```python
from build123d import *

# Parameters (mm, degrees)
SKETCH_1_W           = 67.5
SKETCH_1_H           = 62.5
EXTRUDE_1_DEPTH      = 1.6
SKETCH_2_R           = 1.65
CUT_EXTRUDE_1_DEPTH  = 10
CHAMFER_1_SIZE       = 3
SKETCH_3_R           = 1.65
EXTRUDE_2_DEPTH      = 4
SKETCH_4_R           = 4
CUT_EXTRUDE_2_DEPTH  = 0.8
SKETCH_5_R           = 4.5
EXTRUDE_3_DEPTH      = 6
EXTRUDE_4_DEPTH      = 8
EXTRUDE_5_DEPTH      = 2
CUT_EXTRUDE_4_DEPTH  = 8
EXTRUDE_6_DEPTH      = 2
EXTRUDE_6_DEPTH_BACK = 2
SKETCH_10_R          = 4.5
SKETCH_10_R_2        = 1.65


with BuildPart() as part:
    # 草图1 → 凸台-拉伸1 (new body)
    with BuildSketch(Plane.XY):
        Rectangle(SKETCH_1_W, SKETCH_1_H)
    extrude(amount=EXTRUDE_1_DEPTH)

    # 草图2 → 切除-拉伸1 (cut)
    with BuildSketch(Plane.XY.offset(1.6)):
        with Locations((-22.5, 20)):
            Circle(SKETCH_2_R)
        with Locations((22.5, 20)):
            Circle(SKETCH_2_R)
        with Locations((22.5, -20)):
            Circle(SKETCH_2_R)
        with Locations((-22.5, -20)):
            Circle(SKETCH_2_R)
        Polygon((-30.75, 11.25), (-30.75, -11.25), (-33.75, -14.25), (-33.75, 14.25), align=None)
        Polygon((30.75, 11.25), (30.75, -11.25), (33.75, -14.25), (33.75, 14.25), align=None)
    extrude(amount=-CUT_EXTRUDE_1_DEPTH, mode=Mode.SUBTRACT)

    # 倒角1
    chamfer_1_edges = [part.edges().sort_by_distance(p)[0] for p in [
        (33.75, -31.25, 0.8),
        (-33.75, -31.25, 0.8),
        (-33.75, 31.25, 0.8),
        (33.75, 31.25, 0.8),
    ]]
    chamfer(chamfer_1_edges, length=CHAMFER_1_SIZE)

    # 草图3 → 凸台-拉伸2 (add)
    # profile 1 of 4: a face of its own
    with BuildSketch(Plane(origin=(0, 0, 0), x_dir=(-1, 0, 0), z_dir=(0, 0, -1))):
        Polygon((-19.901923789, 20), (-21.200961894, 22.25), (-23.799038106, 22.25), (-25.098076211, 20), (-23.799038106, 17.75), (-21.200961894, 17.75), align=None)
        with Locations(Location((-22.5, 20, 0), (0, 0, 180))):
            Circle(SKETCH_3_R, mode=Mode.SUBTRACT)
    # profile 2 of 4: a face of its own
    with BuildSketch(Plane(origin=(0, 0, 0), x_dir=(-1, 0, 0), z_dir=(0, 0, -1))):
        Polygon((25.098076211, 20), (23.799038106, 22.25), (21.200961894, 22.25), (19.901923789, 20), (21.200961894, 17.75), (23.799038106, 17.75), align=None)
        with Locations(Location((22.5, 20, 0), (0, 0, 180))):
            Circle(SKETCH_3_R, mode=Mode.SUBTRACT)
    # profile 3 of 4: a face of its own
    with BuildSketch(Plane(origin=(0, 0, 0), x_dir=(-1, 0, 0), z_dir=(0, 0, -1))):
        Polygon((25.098076211, -20), (23.799038106, -17.75), (21.200961894, -17.75), (19.901923789, -20), (21.200961894, -22.25), (23.799038106, -22.25), align=None)
        with Locations(Location((22.5, -20, 0), (0, 0, 180))):
            Circle(SKETCH_3_R, mode=Mode.SUBTRACT)
    # profile 4 of 4: a face of its own
    with BuildSketch(Plane(origin=(0, 0, 0), x_dir=(-1, 0, 0), z_dir=(0, 0, -1))):
        Polygon((-19.901923789, -20), (-21.200961894, -17.75), (-23.799038106, -17.75), (-25.098076211, -20), (-23.799038106, -22.25), (-21.200961894, -22.25), align=None)
        with Locations(Location((-22.5, -20, 0), (0, 0, 180))):
            Circle(SKETCH_3_R, mode=Mode.SUBTRACT)
    extrude(amount=EXTRUDE_2_DEPTH)

    # 草图4 → 切除-拉伸2 (cut)
    with BuildSketch(Plane.XY.offset(1.6)):
        with Locations((-22.5, 20)):
            Circle(SKETCH_4_R)
        with Locations((22.5, 20)):
            Circle(SKETCH_4_R)
        with Locations((22.5, -20)):
            Circle(SKETCH_4_R)
        with Locations((-22.5, -20)):
            Circle(SKETCH_4_R)
    extrude(amount=-CUT_EXTRUDE_2_DEPTH, mode=Mode.SUBTRACT)

    # 草图5 → 凸台-拉伸3 (add)
    # profile 1 of 4: a face of its own
    with BuildSketch(Plane(origin=(0, 0, 0), x_dir=(-1, 0, 0), z_dir=(0, 0, -1))):
        with Locations(Location((-22.5, 20, 0), (0, 0, 180))):
            Circle(SKETCH_5_R)
        Polygon((-21.200961894, 17.75), (-19.901923789, 20), (-21.200961894, 22.25), (-23.799038106, 22.25), (-25.098076211, 20), (-23.799038106, 17.75), align=None, mode=Mode.SUBTRACT)
    # profile 2 of 4: a face of its own
    with BuildSketch(Plane(origin=(0, 0, 0), x_dir=(-1, 0, 0), z_dir=(0, 0, -1))):
        with Locations(Location((22.5, 20, 0), (0, 0, 180))):
            Circle(SKETCH_5_R)
        Polygon((23.799038106, 17.75), (25.098076211, 20), (23.799038106, 22.25), (21.200961894, 22.25), (19.901923789, 20), (21.200961894, 17.75), align=None, mode=Mode.SUBTRACT)
    # profile 3 of 4: a face of its own
    with BuildSketch(Plane(origin=(0, 0, 0), x_dir=(-1, 0, 0), z_dir=(0, 0, -1))):
        with Locations(Location((22.5, -20, 0), (0, 0, 180))):
            Circle(SKETCH_5_R)
        Polygon((23.799038106, -22.25), (25.098076211, -20), (23.799038106, -17.75), (21.200961894, -17.75), (19.901923789, -20), (21.200961894, -22.25), align=None, mode=Mode.SUBTRACT)
    # profile 4 of 4: a face of its own
    with BuildSketch(Plane(origin=(0, 0, 0), x_dir=(-1, 0, 0), z_dir=(0, 0, -1))):
        with Locations(Location((-22.5, -20, 0), (0, 0, 180))):
            Circle(SKETCH_5_R)
        Polygon((-21.200961894, -22.25), (-19.901923789, -20), (-21.200961894, -17.75), (-23.799038106, -17.75), (-25.098076211, -20), (-23.799038106, -22.25), align=None, mode=Mode.SUBTRACT)
    extrude(amount=EXTRUDE_3_DEPTH)

    # 草图6 → 凸台-拉伸4 (add)
    with BuildSketch(Plane(origin=(0, 0, 0), x_dir=(-1, 0, 0), z_dir=(0, 0, -1))):
        Polygon((-30.75, -31.25), (30.75, -31.25), (33.75, -28.25), (33.75, -14.25), (30.75, -11.25), (30.75, 11.25), (33.75, 14.25), (33.75, 28.25), (30.75, 31.25), (-30.75, 31.25), (-33.75, 28.25), (-33.75, 14.25), (-30.75, 11.25), (-30.75, -11.25), (-33.75, -14.25), (-33.75, -28.25), align=None)
        Polygon((-30.335786438, -30.25), (30.335786438, -30.25), (32.75, -27.835786438), (32.75, -14.664213562), (29.75, -11.664213562), (29.75, 11.664213562), (32.75, 14.664213562), (32.75, 27.835786438), (30.335786438, 30.25), (-30.335786438, 30.25), (-32.75, 27.835786438), (-32.75, 14.664213562), (-29.75, 11.664213562), (-29.75, -11.664213562), (-32.75, -14.664213562), (-32.75, -27.835786438), align=None, mode=Mode.SUBTRACT)
    extrude(amount=EXTRUDE_4_DEPTH)

    # 草图8 → 凸台-拉伸5 (add)
    with BuildSketch(Plane(origin=(0, 0, 0), x_dir=(-1, 0, 0), z_dir=(0, 0, -1))):
        with BuildLine():
            Line((-1.5, -11.14955156), (-1.5, -12.157816416))
            ThreePointArc((-1.5, -12.157816416), (0, 12.25), (1.5, -12.157816416))
            Line((1.5, -12.157816416), (1.5, -11.14955156))
            ThreePointArc((1.5, -11.14955156), (0, 11.25), (-1.5, -11.14955156))
        make_face()
    extrude(amount=EXTRUDE_5_DEPTH)

    # 草图9 → 切除-拉伸4 (cut)
    with BuildSketch(Plane(origin=(0, 0, -8), x_dir=(-1, 0, 0), z_dir=(0, 0, -1))):
        Polygon((29.75, 11.664213562), (32.335786438, 14.25), (33.042893219, 13.542893219), (30.75, 11.25), (30.75, -11.25), (33.042893219, -13.542893219), (32.335786438, -14.25), (29.75, -11.664213562), align=None)
        Polygon((-33.042893219, 13.542893219), (-32.335786438, 14.25), (-29.75, 11.664213562), (-29.75, -11.664213562), (-32.335786438, -14.25), (-33.042893219, -13.542893219), (-30.75, -11.25), (-30.75, 11.25), align=None)
    extrude(amount=-CUT_EXTRUDE_4_DEPTH, mode=Mode.SUBTRACT)

    # 草图10 → 凸台-拉伸6 (add, two sides: drawn at the far end of the back side and taken through both)
    # profile 1 of 4: a face of its own
    with BuildSketch(Plane(origin=(0, 0, -6), x_dir=(-1, 0, 0), z_dir=(0, 0, -1)).offset(-EXTRUDE_6_DEPTH_BACK)):
        with Locations(Location((-22.5, -20, 0), (0, 0, 180))):
            Circle(SKETCH_10_R)
        with Locations(Location((-22.5, -20, 0), (0, 0, 180))):
            Circle(SKETCH_10_R_2, mode=Mode.SUBTRACT)
    # profile 2 of 4: a face of its own
    with BuildSketch(Plane(origin=(0, 0, -6), x_dir=(-1, 0, 0), z_dir=(0, 0, -1)).offset(-EXTRUDE_6_DEPTH_BACK)):
        with Locations(Location((22.5, 20, 0), (0, 0, 180))):
            Circle(SKETCH_10_R)
        with Locations(Location((22.5, 20, 0), (0, 0, 180))):
            Circle(SKETCH_10_R_2, mode=Mode.SUBTRACT)
    # profile 3 of 4: a face of its own
    with BuildSketch(Plane(origin=(0, 0, -6), x_dir=(-1, 0, 0), z_dir=(0, 0, -1)).offset(-EXTRUDE_6_DEPTH_BACK)):
        with Locations(Location((-22.5, 20, 0), (0, 0, 180))):
            Circle(SKETCH_10_R)
        with Locations(Location((-22.5, 20, 0), (0, 0, 180))):
            Circle(SKETCH_10_R_2, mode=Mode.SUBTRACT)
    # profile 4 of 4: a face of its own
    with BuildSketch(Plane(origin=(0, 0, -6), x_dir=(-1, 0, 0), z_dir=(0, 0, -1)).offset(-EXTRUDE_6_DEPTH_BACK)):
        with Locations(Location((22.5, -20, 0), (0, 0, 180))):
            Circle(SKETCH_10_R)
        with Locations(Location((22.5, -20, 0), (0, 0, 180))):
            Circle(SKETCH_10_R_2, mode=Mode.SUBTRACT)
    extrude(amount=EXTRUDE_6_DEPTH + EXTRUDE_6_DEPTH_BACK)


solid = part.part
```
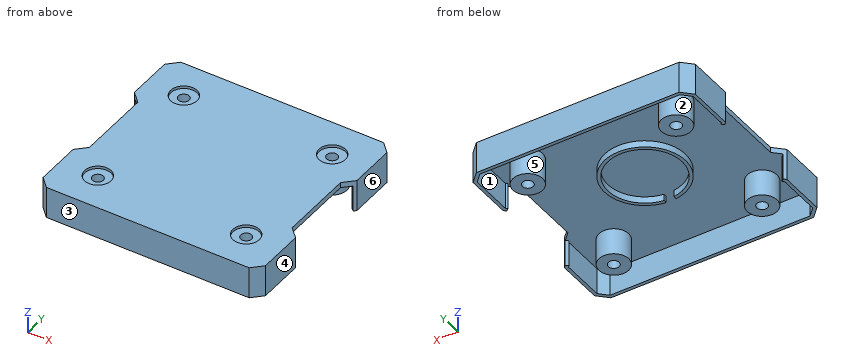
Design review of the part built by this model. Coordinates are the model's own, in mm. Face numbers are marked on the shaded views. A direction names the side the tool comes from. Coordinates: 2 decimals unless noted, no trailing zeros. Write each loop counter-clockwise with the first axis right and the second up, starting at its lowest first coordinate (ties: lowest second). Pieces come first, ordered by that corner, then holes.
1) Insertion check: pin 1 (0.8 mm diameter, centred on y = -11.5, z = -0.5, fed in from +X); pin 2 (18 mm diameter, centred on x = 0, y = 0, fed in from -Z); pin 3 (6.5 mm diameter, centred on x = 22.5, y = 20.5, fed in from +Z); pin 4 (9 mm diameter, centred on x = 23.5, y = -18.5, fed in from +Z). Each pin has a flat end and moves straight along its axis. Give the tip position at first contact, or say it passes through.
2) To check wall thickness, follow L1, parallel to Y at x = 22.5, z = 1.15; L2, parallel to X at y = -20, z = -6.25; L3, parallel to Y at x = -22.5, z = -5.25. State the ranges of each line that lie inside material, in increasing order.
3) Mouldability with a two-part tool opening along X and no side actions: class the marked faces 1, 2, 3 and 4 as +X half, -X half, draft (parallel to the pull), parting line (faces both ways), or undercut.
4) Add section D-D (y = 0). Write out the cut boundary in (x, z).
5) Machinability: for the marked faces 5 and 6, which of the approach directions +Z, -Z, +X, -X, +Y, -Y give a long, thin tool a straight path to every point of the face, cutting with its end or side? Answer none if there is none.
6) Add section A-A (y = -20). State how many separate pieces and enclosed holes the cut face has, plus the area to 3 significant figures.
Check result:
1. pin 1: stops at x = 5.18
1. pin 2: stops at z = 0
1. pin 3: stops at z = 0.8
1. pin 4: stops at z = 1.6
2. L1: y = -31.25 to -24, -16 to 16, 24 to 31.25
2. L2: x = -33.75 to -32.75, -27 to -24.15, -20.85 to -18, 18 to 20.85, 24.15 to 27, 32.75 to 33.75
2. L3: y = -31.25 to -30.25, -24.5 to -21.65, -18.35 to -15.5, 15.5 to 18.35, 21.65 to 24.5, 30.25 to 31.25
3. face 1: undercut
3. face 2: undercut
3. face 3: draft
3. face 4: +X half
4. outline: (-30.75, 0) - (-12.25, 0) - (-12.25, -2) - (-11.25, -2) - (-11.25, 0) - (11.25, 0) - (11.25, -2) - (12.25, -2) - (12.25, 0) - (30.75, 0) - (30.75, 1.6) - (-30.75, 1.6) - close
5. face 5: -Z
5. face 6: +Z, -Z, +X, +Y, -Y
6. separate pieces: 3
6. enclosed holes: 0
6. area: 197 mm2
